```python
from build123d import *

# Parameters (mm, degrees)
BOSS_EXTRUDE1_DEPTH = 8
SKETCH2_W           = 30.98
SKETCH2_H           = 2.54
SKETCH2_W_2         = 41.14
BOSS_EXTRUDE2_DEPTH = 10.5
SKETCH3_R           = 0.5
BOSS_EXTRUDE3_DEPTH = 3


with BuildPart() as part:
    # Sketch1 → Boss-Extrude1 (new body)
    with BuildSketch(Plane(origin=(0, 0, 0), x_dir=(1, 0, 0), z_dir=(0, 1, 0))):
        with BuildLine():
            Line((2, 0), (48.8, 0))
            ThreePointArc((48.8, 0), (50.214213562, 0.585786438), (50.8, 2))
            Line((50.8, 2), (50.8, 20.86))
            ThreePointArc((50.8, 20.86), (50.214213562, 22.274213562), (48.8, 22.86))
            Line((48.8, 22.86), (2, 22.86))
            ThreePointArc((2, 22.86), (0.585786438, 22.274213562), (0, 20.86))
            Line((0, 20.86), (0, 2))
            ThreePointArc((0, 2), (0.585786438, 0.585786438), (2, 0))
        make_face()
    extrude(amount=BOSS_EXTRUDE1_DEPTH)

    # Sketch2 → Boss-Extrude2 (add)
    with BuildSketch(Plane.XZ):
        with Locations((20.49, -1.27)):
            Rectangle(SKETCH2_W, SKETCH2_H)
        with Locations((25.57, -21.59)):
            Rectangle(SKETCH2_W_2, SKETCH2_H)
    extrude(amount=BOSS_EXTRUDE2_DEPTH)

    # Sketch3 → Boss-Extrude3 (add)
    with BuildSketch(Plane.XZ.offset(10.5)):
        with Locations(Location((6.52, -1.27, 0), (0, 0, 270))):
            Circle(SKETCH3_R)
        with Locations(Location((9.06, -1.27, 0), (0, 0, 270))):
            Circle(SKETCH3_R)
        with Locations(Location((11.6, -1.27, 0), (0, 0, 270))):
            Circle(SKETCH3_R)
        with Locations(Location((14.14, -1.27, 0), (0, 0, 270))):
            Circle(SKETCH3_R)
        with Locations(Location((16.68, -1.27, 0), (0, 0, 270))):
            Circle(SKETCH3_R)
        with Locations(Location((19.22, -1.27, 0), (0, 0, 270))):
            Circle(SKETCH3_R)
        with Locations(Location((21.76, -1.27, 0), (0, 0, 270))):
            Circle(SKETCH3_R)
        with Locations(Location((24.3, -1.27, 0), (0, 0, 270))):
            Circle(SKETCH3_R)
        with Locations(Location((26.84, -1.27, 0), (0, 0, 270))):
            Circle(SKETCH3_R)
        with Locations(Location((29.38, -1.27, 0), (0, 0, 270))):
            Circle(SKETCH3_R)
        with Locations(Location((31.92, -1.27, 0), (0, 0, 270))):
            Circle(SKETCH3_R)
        with Locations(Location((34.46, -1.27, 0), (0, 0, 270))):
            Circle(SKETCH3_R)
        with Locations(Location((6.52, -21.59, 0), (0, 0, 90))):
            Circle(SKETCH3_R)
        with Locations(Location((9.06, -21.59, 0), (0, 0, 90))):
            Circle(SKETCH3_R)
        with Locations(Location((11.6, -21.59, 0), (0, 0, 90))):
            Circle(SKETCH3_R)
        with Locations(Location((14.14, -21.59, 0), (0, 0, 90))):
            Circle(SKETCH3_R)
        with Locations(Location((16.68, -21.59, 0), (0, 0, 90))):
            Circle(SKETCH3_R)
        with Locations(Location((19.22, -21.59, 0), (0, 0, 90))):
            Circle(SKETCH3_R)
        with Locations(Location((21.76, -21.59, 0), (0, 0, 90))):
            Circle(SKETCH3_R)
        with Locations(Location((24.3, -21.59, 0), (0, 0, 90))):
            Circle(SKETCH3_R)
        with Locations(Location((26.84, -21.59, 0), (0, 0, 90))):
            Circle(SKETCH3_R)
        with Locations(Location((29.38, -21.59, 0), (0, 0, 90))):
            Circle(SKETCH3_R)
        with Locations(Location((31.92, -21.59, 0), (0, 0, 90))):
            Circle(SKETCH3_R)
        with Locations(Location((34.46, -21.59, 0), (0, 0, 90))):
            Circle(SKETCH3_R)
        with Locations(Location((37, -21.59, 0), (0, 0, 90))):
            Circle(SKETCH3_R)
        with Locations(Location((39.54, -21.59, 0), (0, 0, 90))):
            Circle(SKETCH3_R)
        with Locations(Location((42.08, -21.59, 0), (0, 0, 90))):
            Circle(SKETCH3_R)
        with Locations(Location((44.62, -21.59, 0), (0, 0, 90))):
            Circle(SKETCH3_R)
    extrude(amount=BOSS_EXTRUDE3_DEPTH)


solid = part.part
```
Work out the finished part from the listing and answer in its coordinate system (mm). A direction names the side the tool comes from. Give positions to 0.01 mm unless a question says otherwise; leave off trailing zeros. Loops run counter-clockwise (first coordinate to the right, second up) from the corner with the lowest first, then second, coordinate; pieces in that order, holes last. Notation, with made-up numbers: (-0.75, -29) -> (19.25, -29) arc R16 cw to (19.25, 2) -> close; hole circle Ø4 at (63.5, -35.5). An arc over 180 degrees is marked (long way). Put each result on its own line as item: value. Start each with the question number.
Item 1: The part is cut by section D-D (x = 4). Give the vertices of the cut face in (y, z), then the cut area to 3 significant figures.
Item 2: The part is cut by section A-A (x = 24.3). Give the vertices of the cut face in (y, z), then the cut area to 3 significant figures.
Item 3: Which of the six approach directions +Z, -Z, +X, -X, +Y, -Y give full straight-line access (tool end or side, diameter ignored) to faces 1 (the face through (26, -1, -22.86)), 2 (the face through (19.64, -11.98, -1.54))?
Item 4: Find the intervals of material crossed by L1, parallel to Z at x = 13, y = -2.75; L2, parallel to X at y = -4.5, z = -22; L3, parallel to X at y = -7.75, z = -1, in increasing order. Write a range as [from, to].
Item 5: Each of these flat-tipped pins is pushed along its axis until it touches: P1, Ø1.5, axis at x = 44, y = -6.5, coming from the +Z side; P2, Ø6, axis at y = -4.5, z = -14, coming from the +X side; P3, Ø3, axis at y = -4, z = -1.5, coming from the -X side; P4, Ø2, axis at x = 43, z = -11.5, coming from the -Y side. Where does it stop, or does it pass through?
Item 6: The mould has two halves that part along X. Classify faces 3 (the face through (16.192, -11.979, -1.162)), 4 (the face through (0.57, 3.94, -0.6)), 5 (the face through (25, -1, 0)): released by +X, released by -X, zero draft, split by the parting line, or undercut.
Item 7: The part is cut by section C-C (x = 37). Give the vertices of the cut face in (y, z).
Item 8: The part is cut by section B-B (z = -9.25). Give the vertices of the cut face in (x, y).
Answers below:
1. outline: (0, -22.86) -> (8, -22.86) -> (8, 0) -> (0, 0) -> close
1. area: 183 mm2
2. outline: (-13.5, -22.09) -> (-10.5, -22.09) -> (-10.5, -22.86) -> (8, -22.86) -> (8, 0) -> (-10.5, 0) -> (-10.5, -0.77) -> (-13.5, -0.77) -> (-13.5, -1.77) -> (-10.5, -1.77) -> (-10.5, -2.54) -> (0, -2.54) -> (0, -20.32) -> (-10.5, -20.32) -> (-10.5, -21.09) -> (-13.5, -21.09) -> close
2. area: 242 mm2
3. face 1: -Z, +X, -X, +Y, -Y
3. face 2: -Y
4. L1: [-22.86, -20.32], [-2.54, 0]
4. L2: [5, 46.14]
4. L3: [5, 35.98]
5. P1: z = -20.32
5. P2: through
5. P3: x = 5
5. P4: y = 0
6. face 3: undercut
6. face 4: released by -X
6. face 5: zero draft
7. outline: (-13.5, -22.09) -> (-10.5, -22.09) -> (-10.5, -22.86) -> (8, -22.86) -> (8, 0) -> (0, 0) -> (0, -20.32) -> (-10.5, -20.32) -> (-10.5, -21.09) -> (-13.5, -21.09) -> close
8. outline: (0, 0) -> (50.8, 0) -> (50.8, 8) -> (0, 8) -> close
